Read the model definition and answer for the solid it produces. Units are mm, in the model's axes. Face numbers are marked on the shaded views. Coordinates: 2 decimals unless noted, no trailing zeros. Write each loop counter-clockwise with the first axis right and the second up, starting at its lowest first coordinate (ties: lowest second). Pieces come first, ordered by that corner, then holes. Notation, with made-up numbers: (59.25, -3.5) - (81.25, -3.5) arc R20 cw to (81.25, 30.5) - close; hole circle Ø6 at (89.5, 63). An arc over 180 degrees is marked (long way). Return JSON: item names as keys, results as strings.
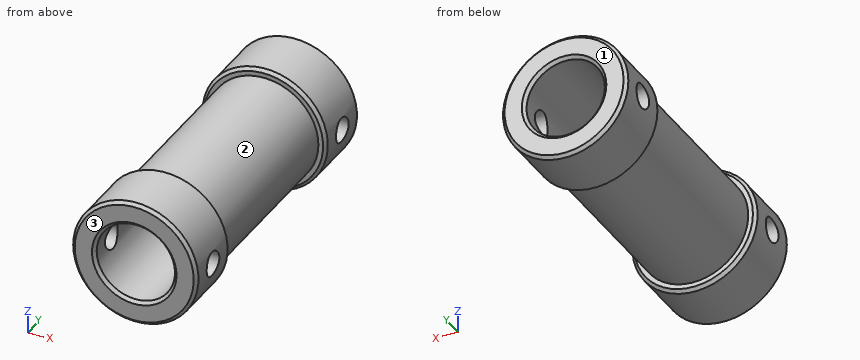
Autodesk Inventor part; units mm, degrees
ref_plane "Work Plane1" through (0, 10, 0) normal (0, 1, 0) x (1, 0, 0)
ref_plane "Work Plane2" through (4, 0, 0) normal (1, 0, 0) x (0, 1, 0)
ref_plane "XZ Plane" through (0, 0, 0) normal (0, 1, 0) x (-1, 0, 0)
sketch "Sketch1" plane through (0, 0, 0) normal (0, 1, 0) x (-1, 0, 0)
  circle A0 centre (0, 0) radius 2.5
  circle A1 centre (0, 0) radius 4
  dimension "d0" = 5
  dimension "d1" = 8
extrude "Extrusion1" add sketch "Sketch1" along normal blind 20
ref_plane "Work Plane1" through (0, 10, 0) normal (0, 1, 0) x (1, 0, 0)
sketch "Sketch2" plane through (0, 10, 0) normal (0, 1, 0) x (1, 0, 0)
  circle A0 centre (0, 0) radius 2.5
  circle A1 centre (0, 0) radius 4
  circle A2 centre (0, 0) radius 3.5
  dimension "d5" = 5
  dimension "d6" = 7
extrude "Extrusion2" cut sketch "Sketch2" along normal mid plane 12 contours A1
chamfer "Chamfer1" distance 0.2 angle 45 4 edges at (4, 0, 0) (4, 4, 0) (4, 16, 0) (4, 20, 0)
chamfer "Chamfer2" distance 0.2 angle 45 2 edges at (2.5, 20, 0) (2.5, 0, 0)
ref_plane "Work Plane2" through (4, 0, 0) normal (1, 0, 0) x (0, 1, 0)
sketch "Sketch3" plane through (4, 0, 0) normal (1, 0, 0) x (0, 1, 0)
  point P0 (0, 0)
  point P1 (2, 0)
  point P2 (18, 0)
  dimension "d15" = 16
  dimension "d16" = 2
hole "Hole1" at (4, 2, 0) at (4, 18, 0) direction (-1, 0, 0) diameter 1.567 end through all
properties part number "Khop_Noi_Truc_5_5"
(1) Determine the mould class of the marked faces 1, 2 and 3 for opening direction Y: +Y half, -Y half, draft (parallel to the pull), parting line (faces both ways), or undercut.
Answer:
{"face 1": "+Y half", "face 2": "undercut", "face 3": "-Y half"}
(2) Flat-ended cylindrical pins translate along their axes: P1, Ø2.5, axis at x = -1, z = -0.5, coming from the +Y side; P2, Ø3, axis at y = 12, z = 3, coming from the -X side. Find the tip coordinate at first contact, or state that the pin passes through.
Answer:
{"P1": "through", "P2": "x = -3.16"}
(3) A cutting plane is placed at C-C (z = 0). State how many separate pieces and enclosed holes the cut face has, and give its area (3 significant figures).
Answer:
{"separate pieces": "6", "enclosed holes": "0", "area": "38.4 mm²"}
(4) A cutting plane is placed at B-B (y = 4.5). Determine the outline of the cut face in (x, z), and give its area (3 significant figures).
Answer:
{"outline": "circle Ø7 at (0, 0); hole circle Ø5 at (0, 0)", "area": "18.8 mm²"}
(5) A cutting plane is placed at D-D (y = 18). Determine the outline of the cut face in (x, z), and give its area (3 significant figures).
Answer:
{"outline": "(-3.92, -0.78) arc R4 ccw to (3.92, -0.78) - (2.37, -0.78) arc R2.5 cw to (-2.37, -0.78) - close; (-3.92, 0.78) - (-2.37, 0.78) arc R2.5 cw to (2.37, 0.78) - (3.92, 0.78) arc R4 ccw to start", "area": "25.9 mm²"}
(6) A cutting plane is placed at A-A (x = 0). Determine the outline of the cut face in (y, z).
Answer:
{"outline": "(0, -3.8) - (0.2, -4) - (3.8, -4) - (4, -3.8) - (4, -3.5) - (16, -3.5) - (16, -3.8) - (16.2, -4) - (19.8, -4) - (20, -3.8) - (20, -2.7) - (19.8, -2.5) - (0.2, -2.5) - (0, -2.7) - close; (0, 2.7) - (0.2, 2.5) - (19.8, 2.5) - (20, 2.7) - (20, 3.8) - (19.8, 4) - (16.2, 4) - (16, 3.8) - (16, 3.5) - (4, 3.5) - (4, 3.8) - (3.8, 4) - (0.2, 4) - (0, 3.8) - close"}
(7) Straight lines are drawn through the part: line 1 (Y direction, x = 2.5, z = 2.75); line 2 (Z direction, x = 0, y = 12.75); line 3 (Z direction, x = -2.25, y = 8). For each, find the intervals that lie inside material, in ascending order. Write a range as from..to.
Answer:
{"line 1": "0..4, 16..20", "line 2": "-3.5..-2.5, 2.5..3.5", "line 3": "-2.68..-1.09, 1.09..2.68"}
